from build123d import *

# Parameters (mm, degrees)
SKETCH1_R               = 12.7
BOSS_EXTRUDE1_DEPTH     = 40.9448
CUT_EXTRUDE1_START      = -11.43
CUT_EXTRUDE1_DEPTH      = 11.43
CUT_EXTRUDE2_DEPTH      = 11.43
CUT_EXTRUDE3_DEPTH      = 48.441216753
CUT_EXTRUDE3_DEPTH_BACK = 48.441216753
SKETCH4_R               = 3.175
SKETCH5_R               = 2.54
CUT_EXTRUDE4_DEPTH      = 35.550013459
BOSS_EXTRUDE2_REACH     = 49.441
BOSS_EXTRUDE3_DEPTH     = 1.27


with BuildPart() as part:
    # Sketch1 → Boss-Extrude1 (new body)
    with BuildSketch(Plane(origin=(0, 0, 0), x_dir=(1, 0, 0), z_dir=(0, 1, 0))):
        with Locations(Location((0, 0, 0), (0, 0, 270))):
            Circle(SKETCH1_R)
    extrude(amount=BOSS_EXTRUDE1_DEPTH)

    # Sketch2 → Cut-Extrude1 (cut)
    with BuildSketch(Plane(origin=(0, 40.9448, 0), x_dir=(1, 0, 0), z_dir=(0, 1, 0)).offset(CUT_EXTRUDE1_START)):
        with BuildLine():
            Line((7.62, 10.16), (7.62, -10.16))
            ThreePointArc((7.62, -10.16), (0, -12.7), (-7.62, -10.16))
            Line((-7.62, -10.16), (-7.62, 10.16))
            ThreePointArc((-7.62, 10.16), (0, 12.7), (7.62, 10.16))
        make_face()
    extrude(amount=CUT_EXTRUDE1_DEPTH, mode=Mode.SUBTRACT)

    # Sketch3 → Cut-Extrude2 (cut)
    with BuildSketch(Plane.XZ):
        with BuildLine():
            Line((-2.54, 12.443407893), (-2.54, -12.443407893))
            ThreePointArc((-2.54, -12.443407893), (0, -12.7), (2.54, -12.443407893))
            Line((2.54, -12.443407893), (2.54, 12.443407893))
            ThreePointArc((2.54, 12.443407893), (0, 12.7), (-2.54, 12.443407893))
        make_face()
        with BuildLine():
            Line((-7.62, 10.16), (-7.62, -10.16))
            ThreePointArc((-7.62, -10.16), (-12.7, 0), (-7.62, 10.16))
        make_face()
        with BuildLine():
            Line((7.62, 10.16), (7.62, -10.16))
            ThreePointArc((7.62, -10.16), (12.7, 0), (7.62, 10.16))
        make_face()
    extrude(amount=-CUT_EXTRUDE2_DEPTH, mode=Mode.SUBTRACT)

    # Sketch4 → Cut-Extrude3 (cut, two sides: drawn at the far end of the back side and taken through both)
    with BuildSketch(Plane(origin=(-7.62, 0, 0), x_dir=(0, 0, -1), z_dir=(1, 0, 0)).offset(-CUT_EXTRUDE3_DEPTH_BACK)):
        with Locations(Location((0, 35.8648, 0), (0, 0, 270))):
            Circle(SKETCH4_R)
        with Locations((0, 5.08)):
            Circle(SKETCH4_R)
        with BuildLine():
            Line((0, 40.9448), (-10.16, 40.9448))
            Line((-10.16, 40.9448), (-10.16, 29.5148))
            Line((-10.16, 29.5148), (-4.264917923, 38.624668677))
            ThreePointArc((-4.264917923, 38.624668677), (-2.427577715, 40.327228312), (0, 40.9448))
        make_face()
        with BuildLine():
            Line((0, 0), (-12.443407893, 0))
            Line((-12.443407893, 0), (-12.443407893, 11.43))
            Line((-12.443407893, 11.43), (-3.796422114, 1.704562379))
            ThreePointArc((-3.796422114, 1.704562379), (-2.080766311, 0.445691901), (0, 0))
        make_face()
    extrude(amount=CUT_EXTRUDE3_DEPTH + CUT_EXTRUDE3_DEPTH_BACK, mode=Mode.SUBTRACT)

    # Sketch5 → Cut-Extrude4 (cut, through all)
    with BuildSketch(Plane(origin=(0, 29.5148, 0), x_dir=(1, 0, 0), z_dir=(0, 1, 0))):
        with Locations(Location((0, 0, 0), (0, 0, 270))):
            Circle(SKETCH5_R)
    extrude(amount=-CUT_EXTRUDE4_DEPTH, mode=Mode.SUBTRACT)

    # Boss-Extrude2: up to this face of the body (flat: up to its plane)
    boss_extrude2_end = Plane(part.part.faces().sort_by_distance((7.62, 29.747941009, 0))[0])
    # Sketch6 → Boss-Extrude2 (add, up to the picked face)
    with BuildSketch(Plane(origin=(-7.62, 0, 0), x_dir=(0, 0, -1), z_dir=(1, 0, 0)), mode=Mode.PRIVATE) as boss_extrude2_sk1:
        Polygon((2.54, 29.5148), (10.16, 29.5148), (10.16, 30.7848), (7.62, 30.7848), align=None)
    boss_extrude2_tool1 = split(extrude(boss_extrude2_sk1.sketch, amount=BOSS_EXTRUDE2_REACH, mode=Mode.PRIVATE), bisect_by=boss_extrude2_end, keep=Keep.BOTH, mode=Mode.PRIVATE)
    add(boss_extrude2_tool1.solids().sort_by(Axis((-7.62, 30.043967, -7.408333), (1, 0, 0)))[0])

    # Sketch7 → Boss-Extrude3 (add)
    with BuildSketch(Plane(origin=(0, 29.5148, 0), x_dir=(1, 0, 0), z_dir=(0, 1, 0))):
        with BuildLine():
            Line((-7.62, 10.16), (7.62, 10.16))
            ThreePointArc((7.62, 10.16), (0, 12.7), (-7.62, 10.16))
        make_face()
    extrude(amount=BOSS_EXTRUDE3_DEPTH)


solid = part.part
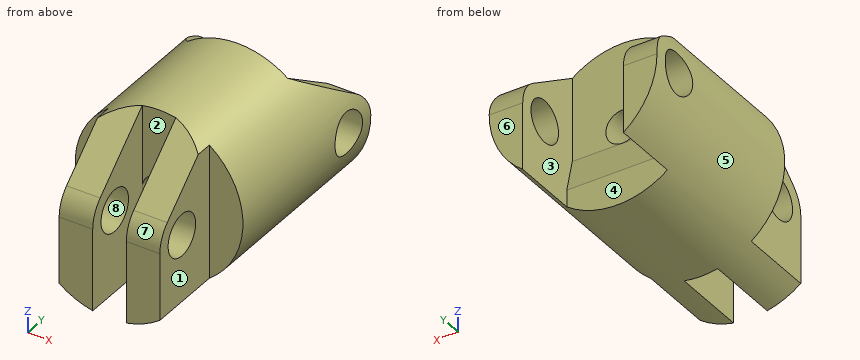
Here's how the part is built. I have some questions about the finished solid (model axes, mm). Face numbers are marked on the shaded views. A direction names the side the tool comes from. Coordinates: 2 decimals unless noted, no trailing zeros. Write each loop counter-clockwise with the first axis right and the second up, starting at its lowest first coordinate (ties: lowest second). Pieces come first, ordered by that corner, then holes.
Item 1: If we mould it in two halves opening along Z, with no side actions, what happens to the marked faces 5, 6, 7 and 8? For each: +Z half, -Z half, draft (parallel to the pull), parting line (faces both ways), or undercut.
Item 2: I want a section at B-B on x = -5.75. Write out the boundary of the cut face in (y, z) (3 decimals), and give its area (3 significant figures).
Item 3: I want a section at A-A on y = 36.5. Write out the boundary of the cut face in (x, z), and give its area (3 significant figures).
Item 4: I want a section at C-C on y = 12. Write out the boundary of the cut face in (x, z).
Item 5: If I drill on line 1 (X direction, y = 7, z = 4.75); line 2 (X direction, y = 31, z = 2); line 3 (Y direction, x = 2.5, z = -10), over which ranges is the centre line in solid material (lowest first)?
Item 6: On a 3-axis mill with a long thin cutter (end or side, diameter ignored), from which of +Z, -Z, +X, -X, +Y, -Y can I reach the whole of each face in a straight line? I mean the marked faces 1, 2, 3 and 4. Say none if no direction works.
Item 7: I want a section at D-D on z = 10.75. Write out the boundary of the cut face in (x, y), and give its area (3 significant figures).
Item 8: Will these pins go through, and if not, where does the flat tip stop? pin 1 (12 mm diameter, centred on x = -7, y = 20, fed in from +Z); pin 2 (1 mm diameter, centred on y = 20.5, z = -6.5, fed in from -X); pin 3 (2 mm diameter, centred on x = -6, z = 4, fed in from +Y); pin 4 (5 mm diameter, centred on y = 35.86, z = 0, fed in from -X).
Findings below:
1. face 5: parting line
1. face 6: draft
1. face 7: +Z half
1. face 8: undercut
2. outline: (0, -11.324) - (30.785, -11.324) - (30.785, -7.62) - (29.515, -2.54) - (29.515, 11.324) - (10.171, 11.324) - (1.705, 3.796) arc R5.08 ccw to (0, 0) - close; hole circle Ø6.35 at (5.08, 0)
2. area: 598 mm2
3. outline: (-12.31, -3.11) arc R12.7 ccw to (-7.62, -10.16) - (-7.62, -3.11) - close; (-12.31, 3.11) - (-7.62, 3.11) - (-7.62, 5.64) - (-11.38, 5.64) arc R12.7 ccw to start; (7.62, -10.16) arc R12.7 ccw to (12.31, -3.11) - (7.62, -3.11) - close; (7.62, 3.11) - (12.31, 3.11) arc R12.7 ccw to (11.38, 5.64) - (7.62, 5.64) - close
3. area: 63.0 mm2
4. outline: circle Ø25.4 at (0, 0); hole circle Ø5.08 at (0, 0)
5. line 1: x = -7.62 to -2.54, 2.54 to 7.62
5. line 2: x = -12.54 to -7.62, 7.62 to 12.54
5. line 3: y = 11.43 to 30.78
6. face 1: +Z, -Z, +X, -Y
6. face 2: +Z, -Z, -Y
6. face 3: +Z, +Y
6. face 4: +Z, -Z, +Y
7. outline: (-6.76, 9.53) - (-2.54, 9.53) - (-2.54, 11.43) - (2.54, 11.43) - (2.54, 9.53) - (6.76, 9.53) - (6.76, 29.51) - (-6.76, 29.51) - close
7. area: 261 mm2
8. pin 1: stops at z = 12.66
8. pin 2: stops at x = -11.19
8. pin 3: stops at y = 29.51
8. pin 4: passes through
